Check sheet for the modelled part. Datum: model origin and axes. Units: mm. A direction names the side the tool comes from. Round coordinates to 2 decimals unless told otherwise and drop trailing zeros. Write each loop counter-clockwise with the first axis right and the second up, starting at its lowest first coordinate (ties: lowest second). Pieces come first, ordered by that corner, then holes.
Item 1: Section check C-C, the plane y = 7.5. Record the cut outline in (x, z).
Item 2: Material ranges on line 1 along X through (y, z) = (6.75, 1.65); line 2 along Y through (x, z) = (-3.5, 2.2); line 3 along Y through (x, z) = (25, 2.1), recorded low to high.
Item 3: Release check for a two-part mould opening along Y. For faces 4 (the cylindrical face through (0.488, 14.287, 1.878)), 5 (the flat face through (-1, 8, 3.81)), 6 (the flat face through (36, 3.81, 2)), 7 (the flat face through (-36, 12.7, 2)) record: pulls with the +Y half, pulls with the -Y half, needs draft (parallel to the pull), parting line crosses it, or undercut.
Item 4: Depth check by flat-ended pin: pin 1 (1.9 mm diameter, centred on y = 9.5, z = 1.5, fed in from +X). Enter the tip coordinate at first touch or a pass-through.
Item 5: Section check B-B, the plane y = 15. Record the cut outline in (x, z), plus the area to 3 significant figures.
Item 6: Set-up check for faces 1 (the flat face through (-36, 3.81, 2)), 2 (the flat face through (36, 12.7, 2)), 3 (the flat face through (-36, 16.51, 2)): record each of +Z, -Z, +X, -X, +Y, -Y from which the full face is reachable in a straight line by a thin tool's end or side.
Item 7: Section check A-A, the plane z = 3. Record the cut outline in (x, y), plus the area to 3 significant figures.
Item 8: Section check D-D, the plane x = -1.5. Record the cut outline in (y, z).
from build123d import *

# Parameters (mm, degrees)
BOSS_EXTRUDE1_DEPTH = 3.81


with BuildPart() as part:
    # Sketch1 → Boss-Extrude1 (new body)
    with BuildSketch(Plane.XY):
        with BuildLine():
            Line((-38.1, 0), (38.1, 0))
            Line((38.1, 0), (38.1, 3.81))
            Line((38.1, 3.81), (34.29, 3.81))
            Line((34.29, 3.81), (34.29, 12.7))
            Line((34.29, 12.7), (38.1, 12.7))
            Line((38.1, 12.7), (38.1, 16.711046713))
            Line((38.1, 16.711046713), (34.29, 16.711046713))
            ThreePointArc((34.29, 16.711046713), (0.006816557, 14.285295283), (-34.29, 16.51))
            Line((-34.29, 16.51), (-38.1, 16.51))
            Line((-38.1, 16.51), (-38.1, 12.7))
            Line((-38.1, 12.7), (-34.29, 12.7))
            Line((-34.29, 12.7), (-34.29, 3.81))
            Line((-34.29, 3.81), (-38.1, 3.81))
            Line((-38.1, 3.81), (-38.1, 0))
        make_face()
    extrude(amount=BOSS_EXTRUDE1_DEPTH)


solid = part.part
Values found:
1. outline: (-34.29, 0) - (34.29, 0) - (34.29, 3.81) - (-34.29, 3.81) - close
2. line 1: x = -34.29 to 34.29
2. line 2: y = 0 to 14.3
2. line 3: y = 0 to 15.59
3. face 4: pulls with the +Y half
3. face 5: needs draft
3. face 6: undercut
3. face 7: undercut
4. pin 1: stops at x = 34.29
5. outline: (-38.1, 0) - (-19.79, 0) - (-19.79, 3.81) - (-38.1, 3.81) - close; (18.32, 0) - (38.1, 0) - (38.1, 3.81) - (18.32, 3.81) - close
5. area: 145 mm2
6. face 1: +Z, -Z, -X
6. face 2: +Z, -Z, +X
6. face 3: +Z, -Z, -X, +Y
7. outline: (-38.1, 0) - (38.1, 0) - (38.1, 3.81) - (34.29, 3.81) - (34.29, 12.7) - (38.1, 12.7) - (38.1, 16.71) - (34.29, 16.71) arc R254 cw to (-34.29, 16.51) - (-38.1, 16.51) - (-38.1, 12.7) - (-34.29, 12.7) - (-34.29, 3.81) - (-38.1, 3.81) - close
7. area: 1,090 mm2
8. outline: (0, 0) - (14.29, 0) - (14.29, 3.81) - (0, 3.81) - close
